Read the model definition and answer for the solid it produces. Units are mm, in the model's axes. Round coordinates to 2 decimals unless told otherwise and drop trailing zeros. Loops run counter-clockwise (first coordinate to the right, second up) from the corner with the lowest first, then second, coordinate; pieces in that order, holes last. Notation, with made-up numbers: M -23,14 L 28,14 A17 cw 28,34 Z; hole C 23.5,-32 d6. An arc over 180 degrees is marked long. Answer as CSV lines item,"result".
```python
from build123d import *

# Parameters (mm, degrees)
EXTRUDE_1_DEPTH     = 10
SKETCH_2_R          = 92.5
CUT_EXTRUDE_1_DEPTH = 10


with BuildPart() as part:
    # 草图1 → 凸台-拉伸1 (new body)
    with BuildSketch(Plane(origin=(0, 0, 0), x_dir=(1, 0, 0), z_dir=(0, 1, 0))):
        Polygon((0, 0), (700, 0), (760, 103.923048454), (410, 710.140831103), (290, 710.140831103), (-60, 103.923048454), align=None)
    extrude(amount=EXTRUDE_1_DEPTH)

    # 草图2 → 切除-拉伸1 (cut)
    with BuildSketch(Plane(origin=(0, 10, 0), x_dir=(1, 0, 0), z_dir=(0, 1, 0))):
        with Locations(Location((56.602540378, 101.961524227, 0), (0, 0, 270))):
            Circle(SKETCH_2_R)
        with Locations(Location((643.397459622, 101.961524227, 0), (0, 0, 270))):
            Circle(SKETCH_2_R)
        with Locations(Location((350, 610.140831103, 0), (0, 0, 270))):
            Circle(SKETCH_2_R)
    extrude(amount=-CUT_EXTRUDE_1_DEPTH, mode=Mode.SUBTRACT)


solid = part.part
```
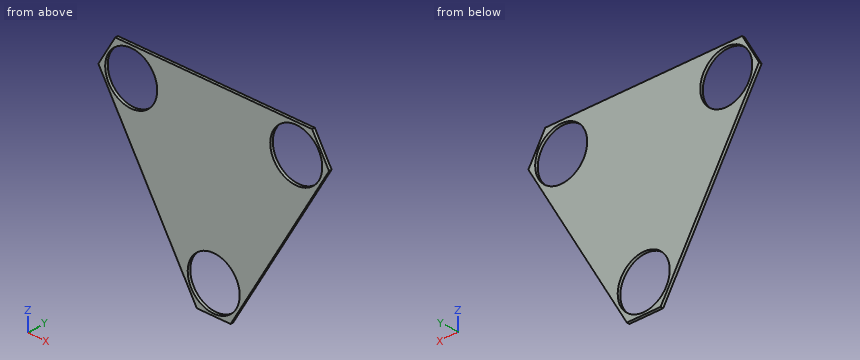
1) Find section A-A, the plane x = 350. Give the vertices of the cut face in (y, z).
Evaluation:
outline,"M 0,-710.14 L 10,-710.14 L 10,-702.64 L 0,-702.64 Z; M 0,-517.64 L 10,-517.64 L 10,0 L 0,0 Z"
2) Find section D-D, the plane y = 5.5. Give the vertices of the cut face in (x, z).
Evaluation:
outline,"M -60,-103.92 L 290,-710.14 L 410,-710.14 L 760,-103.92 L 700,0 L 0,0 Z; hole C 56.6,-101.96 d185; hole C 350,-610.14 d185; hole C 643.4,-101.96 d185"
3) Straight lines are drawn through the part: line 1 (X direction, y = 2, z = -180); line 2 (X direction, y = 6.25, z = -139); line 3 (X direction, y = 3, z = -663). For each, find the intervals that lie inside material, in ascending order.
Evaluation:
line 1,"x = -16.08 to 6.94, 106.26 to 593.74, 693.06 to 716.08"
line 2,"x = -39.75 to -28.16, 141.36 to 558.64, 728.16 to 739.75"
line 3,"x = 262.78 to 274.09, 425.91 to 437.22"
4) Find section C-C, the plane z = -607.5. Give the vertices of the cut face in (x, y), then the cut area to 3 significant figures.
Evaluation:
outline,"M 230.74,0 L 257.54,0 L 257.54,10 L 230.74,10 Z; M 442.46,0 L 469.26,0 L 469.26,10 L 442.46,10 Z"
area,"536 mm^2"
5) Each of these flat-tipped pins is pushed along its axis until it touches: P1, Ø1, axis at y = 5.5, z = -91.5, coming from the -X side; P2, Ø4, axis at y = 4, z = -260, coming from the -X side; P3, Ø6, axis at y = 5.5, z = -590, coming from the -X side. Where does it stop, or does it pass through?
Evaluation:
P1,"stops at x = -53.12"
P2,"stops at x = 28.96"
P3,"stops at x = 218.9"
6) Find section B-B, the plane z = -151.5. Give the vertices of the cut face in (x, y), then the cut area to 3 significant figures.
Evaluation:
outline,"M -32.53,0 L -21.51,0 L -21.51,10 L -32.53,10 Z; M 134.72,0 L 565.28,0 L 565.28,10 L 134.72,10 Z; M 721.51,0 L 732.53,0 L 732.53,10 L 721.51,10 Z"
area,"4,530 mm^2"
